Geometry check sheet. Reference: the model listing, model coordinates, mm. Face numbers are marked on the shaded views. A direction names the side the tool comes from. Round coordinates to 2 decimals unless told otherwise and drop trailing zeros. Write each loop counter-clockwise with the first axis right and the second up, starting at its lowest first coordinate (ties: lowest second). Pieces come first, ordered by that corner, then holes.
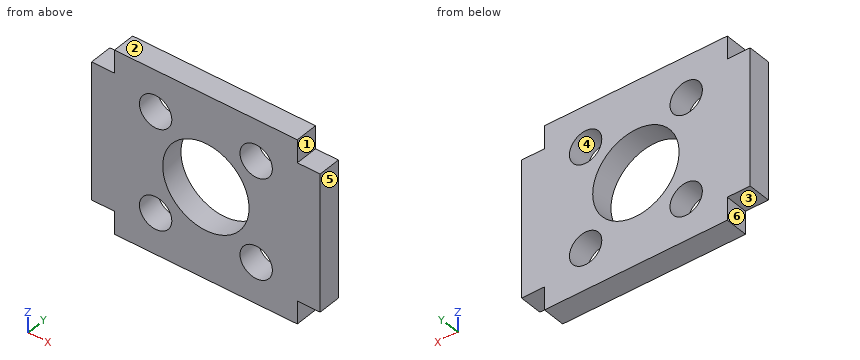
from build123d import *

# Parameters (mm, degrees)
BOSS_EXTRUDE1_DEPTH   = 3.175
SKETCH2_R             = 6
CUT_EXTRUDE1_DEPTH    = 4.175
F_8_CLEARANCE_HOLE1_D = 4.4958


with BuildPart() as part:
    # Sketch1 → Boss-Extrude1 (new body)
    with BuildSketch(Plane(origin=(0, 0, 0), x_dir=(1, 0, 0), z_dir=(0, 1, 0))):
        Polygon((-12.7, 9.525), (-15.875, 9.525), (-15.875, -9.525), (-12.7, -9.525), (-12.7, -12.7), (12.7, -12.7), (12.7, -9.525), (15.875, -9.525), (15.875, 9.525), (12.7, 9.525), (12.7, 12.7), (-12.7, 12.7), align=None)
    extrude(amount=BOSS_EXTRUDE1_DEPTH)

    # Sketch2 → Cut-Extrude1 (cut, through all)
    with BuildSketch(Plane(origin=(0, 3.175, 0), x_dir=(1, 0, 0), z_dir=(0, 1, 0))):
        Circle(SKETCH2_R)
    extrude(amount=-CUT_EXTRUDE1_DEPTH, mode=Mode.SUBTRACT)

    # #8 Clearance Hole1 (through all)
    with Locations(Plane(origin=(0, 3.175, 0), x_dir=(1, 0, 0), z_dir=(0, 1, 0))):
        with Locations((-6.985, 6.985), (6.985, 6.985), (6.985, -6.985), (-6.985, -6.985)):
            Hole(F_8_CLEARANCE_HOLE1_D / 2)


solid = part.part
1. Release check for a two-part mould opening along X. For the marked faces 3, 4, 5 and 6 record: +X half, -X half, draft (parallel to the pull), parting line (faces both ways), or undercut.
2. Section check D-D (y = 0.7). Record the cut outline in (x, z) (3 decimals).
3. Section check B-B (z = 0). Record the cut outline in (x, y) (3 decimals).
4. Depth check by flat-ended pin: pin 1 Ø1 at (y, z) = (2, -11) entering from +X; pin 2 Ø7 at (x, z) = (6.985, 6.985) entering from +Y (3 decimals); pin 3 Ø1 at (y, z) = (1.5, -11.5) entering from -X; pin 4 Ø3.5 at (x, z) = (-6.985, -6.985) entering from +Y. Enter the tip coordinate at first touch or a pass-through.
5. Section check C-C (z = -7.75). Record the cut outline in (x, y) (3 decimals).
6. Scan lines: line 1 along X through (y, z) = (0.4, -7) (3 decimals); line 2 along Z through (x, y) = (7, 2.4); line 3 along X through (y, z) = (1.1, 7.75) (3 decimals). Record each from-to range of solid material in increasing order.
7. Access from +Z, -Z, +X, -X, +Y, -Y to the whole of each face (thin tool, end or side, straight path). Record for the marked faces 1 and 2.
8. Section check A-A (x = 0). Record the cut outline in (y, z) (3 decimals), plus the area to 3 significant figures.
Results below:
1. face 3: draft
1. face 4: undercut
1. face 5: +X half
1. face 6: -X half
2. outline: (-15.875, -9.525) - (-12.7, -9.525) - (-12.7, -12.7) - (12.7, -12.7) - (12.7, -9.525) - (15.875, -9.525) - (15.875, 9.525) - (12.7, 9.525) - (12.7, 12.7) - (-12.7, 12.7) - (-12.7, 9.525) - (-15.875, 9.525) - close; hole circle Ø4.496 at (-6.985, -6.985); hole circle Ø4.496 at (-6.985, 6.985); hole circle Ø12 at (0, 0); hole circle Ø4.496 at (6.985, -6.985); hole circle Ø4.496 at (6.985, 6.985)
3. outline: (-15.875, 0) - (-6, 0) - (-6, 3.175) - (-15.875, 3.175) - close; (6, 0) - (15.875, 0) - (15.875, 3.175) - (6, 3.175) - close
4. pin 1: stops at x = 12.7
4. pin 2: stops at y = 3.175
4. pin 3: stops at x = -12.7
4. pin 4: passes through
5. outline: (-15.875, 0) - (-9.099, 0) - (-9.099, 3.175) - (-15.875, 3.175) - close; (-4.871, 0) - (4.871, 0) - (4.871, 3.175) - (-4.871, 3.175) - close; (9.099, 0) - (15.875, 0) - (15.875, 3.175) - (9.099, 3.175) - close
6. line 1: x = -15.875 to -9.233, -4.737 to 4.737, 9.233 to 15.875
6. line 2: z = -12.7 to -9.23, -4.74 to 4.74, 9.23 to 12.7
6. line 3: x = -15.875 to -9.099, -4.871 to 4.871, 9.099 to 15.875
7. face 1: +Z, +X, +Y, -Y
7. face 2: +Z, +X, -X, +Y, -Y
8. outline: (0, -12.7) - (3.175, -12.7) - (3.175, -6) - (0, -6) - close; (0, 6) - (3.175, 6) - (3.175, 12.7) - (0, 12.7) - close
8. area: 42.5 mm2
